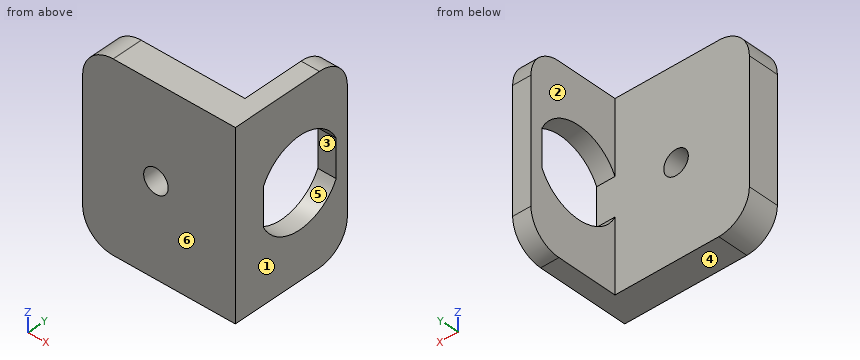
```python
from build123d import *

# Parameters (mm, degrees)
BOSS_EXTRUDE1_DEPTH     = 38.1
F_1_4_20_TAPPED_HOLE1_D = 5.1054
CUT_EXTRUDE1_DEPTH      = 32.75
FILLET1_R               = 6.35


with BuildPart() as part:
    # Sketch1 → Boss-Extrude1 (new body)
    with BuildSketch(Plane.XY):
        Polygon((0, 0), (0, 25.4), (-3.81, 25.4), (-3.81, 6.35), (-31.75, 6.35), (-31.75, 0), align=None)
    extrude(amount=BOSS_EXTRUDE1_DEPTH)

    # 1/4-20 Tapped Hole1 (through all)
    with Locations(Plane(origin=(0, 6.35, 0), x_dir=(1, 0, 0), z_dir=(0, 1, 0))):
        with Locations((-16.51, -19.05)):
            Hole(F_1_4_20_TAPPED_HOLE1_D / 2)

    # Sketch4 → Cut-Extrude1 (cut, through all)
    with BuildSketch(Plane(origin=(0, 0, 0), x_dir=(0, 0, -1), z_dir=(1, 0, 0))):
        with BuildLine():
            Line((-22.982901092, 22.86), (-15.117098908, 22.86))
            ThreePointArc((-15.117098908, 22.86), (-9.906, 14.605), (-15.117098908, 6.35))
            Line((-15.117098908, 6.35), (-22.982901092, 6.35))
            ThreePointArc((-22.982901092, 6.35), (-28.194, 14.605), (-22.982901092, 22.86))
        make_face()
    extrude(amount=-CUT_EXTRUDE1_DEPTH, mode=Mode.SUBTRACT)

    # Fillet1
    fillet1_edges = [part.edges().sort_by_distance(p)[0] for p in [
        (-1.905, 25.4, 38.1),
        (-31.75, 3.175, 38.1),
        (-31.75, 3.175, 0),
        (-1.905, 25.4, 0),
    ]]
    fillet(fillet1_edges, radius=FILLET1_R)


solid = part.part
```
Input: part model. Units: mm. Frame: model coordinates. Face numbers are marked on the shaded views. A direction names the side the tool comes from. Give positions to 0.01 mm unless a question says otherwise; leave off trailing zeros. Order: outer loops, then holes, each group sorted by start corner. A loop starts at its lowest first (then second) coordinate and runs counter-clockwise, first axis right, second up. Notation, with made-up numbers: (1, 3.25) -> (37, 3.25) arc R14 cw to (37, 17.25) -> close; hole circle Ø4 at (87.5, -15). An arc over 180 degrees is marked (long way). Write each question's results on one line, items separated by ' | '. Start each with the question number.
Item 1: Cut plane B-B on z = 19.05. Return the cut outline in (x, y).
Item 2: Cut plane C-C on y = 16.25. Return the cut outline in (x, z).
Item 3: Line query: line 1 (X direction, y = 4.25, z = 19.05); line 2 (Y direction, x = -3, z = 19); line 3 (Z direction, x = -16.51, y = 4.75). Output: solid intervals per line, ascending.
Item 4: Mould query, pull axis Z, two halves, no side actions, for the marked faces 4, 5 and 6. Classes: pulls with the +Z half, pulls with the -Z half, needs draft (parallel to the pull), parting line crosses it, or undercut.
Item 5: Contact query for flat-ended pins moving along their axis: P1, Ø9.5, axis at x = -20.5, z = 17.5, coming from the +Y side; P2, Ø6, axis at y = 12.5, z = 24, coming from the +X side; P3, Ø15, axis at y = 17.5, z = 10, coming from the -X side. Output: stop coordinate, or through.
Item 6: Cut plane D-D on z = 25. Return the cut outline in (x, y).
Item 7: Cut plane A-A on x = -16.51. Return the cut outline in (y, z).
Item 8: Set-up query: the marked faces 1, 2 and 3. Return all of +Z, -Z, +X, -X, +Y, -Y with unobstructed straight access to the full face (end or side cutting, diameter ignored); none if empty.
Established:
1) outline: (-31.75, 0) -> (-19.06, 0) -> (-19.06, 6.35) -> (-31.75, 6.35) -> close; (-13.96, 0) -> (0, 0) -> (0, 6.35) -> (-13.96, 6.35) -> close; (-3.81, 22.86) -> (0, 22.86) -> (0, 25.4) -> (-3.81, 25.4) -> close
2) outline: (-3.81, 0) -> (0, 0) -> (0, 10.06) -> (-3.81, 10.06) -> close; (-3.81, 28.04) -> (0, 28.04) -> (0, 38.1) -> (-3.81, 38.1) -> close
3) line 1: -31.75 to -19.06, -13.96 to 0 | line 2: 0 to 6.35, 22.86 to 25.4 | line 3: 0 to 16.5, 21.6 to 38.1
4) face 4: pulls with the -Z half | face 5: undercut | face 6: needs draft
5) P1: y = 6.35 | P2: through | P3: x = -3.81
6) outline: (-31.75, 0) -> (0, 0) -> (0, 7.66) -> (-3.81, 7.66) -> (-3.81, 6.35) -> (-31.75, 6.35) -> close; (-3.81, 21.55) -> (0, 21.55) -> (0, 25.4) -> (-3.81, 25.4) -> close
7) outline: (0, 0) -> (6.35, 0) -> (6.35, 16.5) -> (0, 16.5) -> close; (0, 21.6) -> (6.35, 21.6) -> (6.35, 38.1) -> (0, 38.1) -> close
8) face 1: +Z, -Z, +X, +Y, -Y | face 2: +Z, -Z, -X, +Y | face 3: +X, -X
